from build123d import *

# Parameters (mm, degrees)
SKETCH1_R           = 28
SKETCH1_R_2         = 26
BOSS_EXTRUDE1_DEPTH = 55
SKETCH2_R           = 28
BOSS_EXTRUDE2_DEPTH = 1.5
SKETCH3_R           = 10
BOSS_EXTRUDE3_DEPTH = 90


with BuildPart() as part:
    # Sketch1 → Boss-Extrude1 (new body)
    with BuildSketch(Plane.XY):
        Circle(SKETCH1_R)
        Circle(SKETCH1_R_2, mode=Mode.SUBTRACT)
    extrude(amount=BOSS_EXTRUDE1_DEPTH)

    # Sketch2 → Boss-Extrude2 (add)
    with BuildSketch(Plane.XY.offset(55)):
        Circle(SKETCH2_R)
    extrude(amount=BOSS_EXTRUDE2_DEPTH)

    # Sketch3 → Boss-Extrude3 (add)
    with BuildSketch(Plane(origin=(0, 0, 55), x_dir=(-1, 0, 0), z_dir=(0, 0, -1))):
        Circle(SKETCH3_R)
    extrude(amount=BOSS_EXTRUDE3_DEPTH)


solid = part.part
Verification items for the finished model (mm, model axes). A direction names the side the tool comes from. Give positions to 0.01 mm unless a question says otherwise; leave off trailing zeros. Write each loop counter-clockwise with the first axis right and the second up, starting at its lowest first coordinate (ties: lowest second). Pieces come first, ordered by that corner, then holes. Notation, with made-up numbers: M -22.75,-18.75 L 16.25,-18.75 A27 ccw 16.25,14.25 Z; hole C 55.25,-11.75 d8. An arc over 180 degrees is marked long. Use CSV: the item, a comma, the result in double quotes.
1) Access from +Z, -Z, +X, -X, +Y, -Y to the whole of each face (thin tool, end or side, straight path). Record for faces 4 (the face through (2.17, -9.76, 10.63)), 5 (the face through (0, 0, 56.5)).
Final values:
face 4,"-Z"
face 5,"+Z, +X, -X, +Y, -Y"
2) Cross-section at C-C (z = 36). Enter the section's corners in (x, y), plus the area to 3 significant figures.
Final values:
outline,"C 0,0 d56; C 0,0 d20; hole C 0,0 d52"
area,"653 mm²"
3) Cross-section at A-A (y = 0). Enter the section's corners in (x, z).
Final values:
outline,"M -28,0 L -26,0 L -26,55 L -10,55 L -10,-35 L 10,-35 L 10,55 L 26,55 L 26,0 L 28,0 L 28,56.5 L -28,56.5 Z"
4) Cross-section at D-D (z = -10.5). Enter the section's corners in (x, y).
Final values:
outline,"C 0,0 d20"
5) Release check for a two-part mould opening along X. For faces 1 (the face through (25.865, -10.724, 27.854)), 2 (the face through (11, 0, 55)), 3 (the face through (0, 0, -35)) record: released by +X, released by -X, zero draft, split by the parting line, or undercut.
Final values:
face 1,"split by the parting line"
face 2,"undercut"
face 3,"zero draft"
6) Material ranges on line 1 along Y through (x, z) = (0, 25); line 2 along Y through (x, z) = (-5.5, 32); line 3 along Z through (x, y) = (-14, -8), recorded low to high.
Final values:
line 1,"-28 to -26, -10 to 10, 26 to 28"
line 2,"-27.45 to -25.41, -8.35 to 8.35, 25.41 to 27.45"
line 3,"55 to 56.5"
7) Go/stop test with flat-tipped pins: pin 1 Ø1.5 at (x, z) = (-19, 26.5) entering from -Y; pin 2 Ø2 at (x, z) = (18.5, 28) entering from -Y; pin 3 Ø8 at (x, z) = (16.5, 5) entering from +Y. Record where each tip stops, or that it passes through.
Final values:
pin 1,"y = -21.24"
pin 2,"y = -21.86"
pin 3,"y = 25.05"
